from build123d import *

# Parameters (mm, degrees)
F0_R        = 2.25
F1_DEPTH    = 1.9
F2_T1_DEPTH = 34.4776428685


# Not quite as in the source:
# - a fillet or chamfer that OpenCascade refuses, or shapes differently, is made with other operations: its cross-section is extruded or revolved along the edge and cut away or added


with BuildPart() as f1:
    # F0 (on Front) → F1 (new body)
    with BuildSketch(Plane.XZ):
        with BuildLine():
            Line((0, -33), (0, -5))
            ThreePointArc((0, -5), (-1.4644660941, -1.4644660941), (-5, 0))
            Line((-5, 0), (-11, 0))
            ThreePointArc((-11, 0), (-14.5355339059, -1.4644660941), (-16, -5))
            Line((-16, -5), (-16, -9))
            ThreePointArc((-16, -9), (-17.4644660941, -12.5355339059), (-21, -14))
            Line((-21, -14), (-51.25, -14))
            ThreePointArc((-51.25, -14), (-54.7855339059, -15.4644660941), (-56.25, -19))
            Line((-56.25, -19), (-56.25, -53))
            ThreePointArc((-56.25, -53), (-54.7855339059, -56.5355339059), (-51.25, -58))
            Line((-51.25, -58), (-37.5, -58))
            ThreePointArc((-37.5, -58), (-33.9644660941, -56.5355339059), (-32.5, -53))
            Line((-32.5, -53), (-32.5, -43))
            Line((-32.5, -43), (-32.5, -38))
            Line((-32.5, -38), (-27.5, -38))
            Line((-27.5, -38), (-5, -38))
            ThreePointArc((-5, -38), (-1.4644660941, -36.5355339059), (0, -33))
        make_face()
        with BuildLine():
            Line((-52.25, -47.125), (-52.25, -24.875))
            ThreePointArc((-52.25, -24.875), (-51.7008252147, -23.5491747853), (-50.375, -23))
            ThreePointArc((-50.375, -23), (-49.0491747853, -23.5491747853), (-48.5, -24.875))
            Line((-48.5, -24.875), (-48.5, -47.125))
            ThreePointArc((-48.5, -47.125), (-49.0491747853, -48.4508252147), (-50.375, -49))
            ThreePointArc((-50.375, -49), (-51.7008252147, -48.4508252147), (-52.25, -47.125))
        make_face(mode=Mode.SUBTRACT)
        with BuildLine():
            Line((-41.25, -47.125), (-41.25, -24.875))
            ThreePointArc((-41.25, -24.875), (-40.7008252147, -23.5491747853), (-39.375, -23))
            ThreePointArc((-39.375, -23), (-38.0491747853, -23.5491747853), (-37.5, -24.875))
            Line((-37.5, -24.875), (-37.5, -47.125))
            ThreePointArc((-37.5, -47.125), (-38.0491747853, -48.4508252147), (-39.375, -49))
            ThreePointArc((-39.375, -49), (-40.7008252147, -48.4508252147), (-41.25, -47.125))
        make_face(mode=Mode.SUBTRACT)
        with Locations((-9, -33)):
            Circle(F0_R, mode=Mode.SUBTRACT)
        with Locations((-9, -9)):
            Circle(F0_R, mode=Mode.SUBTRACT)
    extrude(amount=F1_DEPTH)

    # F2: fillet of radius 3 on 1 edges, made by hand

    # F2_s2 → F2_t1 (cut)
    with BuildSketch(Plane.YZ.offset(-32.5)):
        with BuildLine():
            ThreePointArc((-1.9, -38), (-0.5200806465, -36.8971371542), (0, -35.2089428526))
            Line((0, -35.2089428526), (0, -38))
            Line((0, -38), (-1.9, -38))
        make_face()
    extrude(amount=F2_T1_DEPTH, mode=Mode.SUBTRACT)


solid = f1.part
Read the model definition and answer for the solid it produces. Units are mm, in the model's axes. A direction names the side the tool comes from. Round coordinates to 2 decimals unless told otherwise and drop trailing zeros. Write each loop counter-clockwise with the first axis right and the second up, starting at its lowest first coordinate (ties: lowest second). Pieces come first, ordered by that corner, then holes.
1. The part is cut by section A-A, the plane z = -30. Determine the outline of the cut face in (x, y).
2. The part is cut by section D-D, the plane z = -37. Determine the outline of the cut face in (x, y), then the cut area to 3 significant figures.
3. Given pin 1 Ø0.6 at (y, z) = (-1, -32) entering from +X, flat-ended and moving along its own axis, determine where the tip first touches the part or whether it passes through.
4. Straight lines are drawn through the part: L1, parallel to X at y = -0.75, z = -41.5; L2, parallel to X at y = -1.3, z = -33; L3, parallel to Z at x = -9, y = -1.05. For each, find the intervals that lie inside material, in ascending order.
5. Which of the six approach directions +Z, -Z, +X, -X, +Y, -Y give full straight-line access (tool end or side, diameter ignored) to faces 1 (the face through (-16, -1, -7)), 2 (the face through (-16.731, -0.534, -36.918)), 3 (the face through (-37.5, -1, -36)), 4 (the face through (-44, -1, -58))?
6. The part is cut by section B-B, the plane y = -0.5. Determine the outline of the cut face in (x, z) (3 decimals).
7. Determine the mould class of faces 5 (the face through (-14, -1, -1)), 6 (the face through (-36, -1, -14)), 7 (the face through (-10.66, -0.94, -7.48)) for opening direction X: pulls with the +X half, pulls with the -X half, needs draft (parallel to the pull), parting line crosses it, or undercut.
8. The part is cut by section C-C, the plane x = -26. Determine the outline of the cut face in (y, z), then the cut area to 3 significant figures.
Values:
1. outline: (-56.25, -1.9) - (-52.25, -1.9) - (-52.25, 0) - (-56.25, 0) - close; (-48.5, -1.9) - (-41.25, -1.9) - (-41.25, 0) - (-48.5, 0) - close; (-37.5, -1.9) - (0, -1.9) - (0, 0) - (-37.5, 0) - close
2. outline: (-56.25, -1.9) - (-52.25, -1.9) - (-52.25, 0) - (-56.25, 0) - close; (-48.5, -1.9) - (-41.25, -1.9) - (-41.25, 0) - (-48.5, 0) - close; (-37.5, -1.9) - (-2, -1.9) - (-2, -0.59) - (-32.5, -0.59) - (-32.5, 0) - (-37.5, 0) - close
2. area: 70.7 mm2
3. pin 1: stops at x = 0
4. L1: x = -56.25 to -52.25, -48.5 to -41.25, -37.5 to -32.5
4. L2: x = -56.25 to -52.25, -48.5 to -41.25, -37.5 to -11.25, -6.75 to 0
4. L3: z = -37.49 to -35.25, -30.75 to -11.25, -6.75 to 0
5. face 1: +Z, -X, +Y, -Y
5. face 2: -Z, +X, +Y
5. face 3: +Y, -Y
5. face 4: -Z, +X, -X, +Y, -Y
6. outline: (-56.25, -53) arc R5 ccw to (-51.25, -58) - (-37.5, -58) arc R5 ccw to (-32.5, -53) - (-32.5, -36.867) - (-1.831, -36.867) arc R5 ccw to (0, -33) - (0, -5) arc R5 ccw to (-5, 0) - (-11, 0) arc R5 ccw to (-16, -5) - (-16, -9) arc R5 cw to (-21, -14) - (-51.25, -14) arc R5 ccw to (-56.25, -19) - close; hole (-52.25, -47.125) arc R1.875 ccw to (-48.5, -47.125) - (-48.5, -24.875) arc R1.875 ccw to (-52.25, -24.875) - close; hole (-41.25, -47.125) arc R1.875 ccw to (-37.5, -47.125) - (-37.5, -24.875) arc R1.875 ccw to (-41.25, -24.875) - close; hole circle Ø4.5 at (-9, -33); hole circle Ø4.5 at (-9, -9)
7. face 5: pulls with the -X half
7. face 6: needs draft
7. face 7: undercut
8. outline: (-1.9, -38) arc R3 ccw to (0, -35.21) - (0, -14) - (-1.9, -14) - close
8. area: 44.1 mm2
